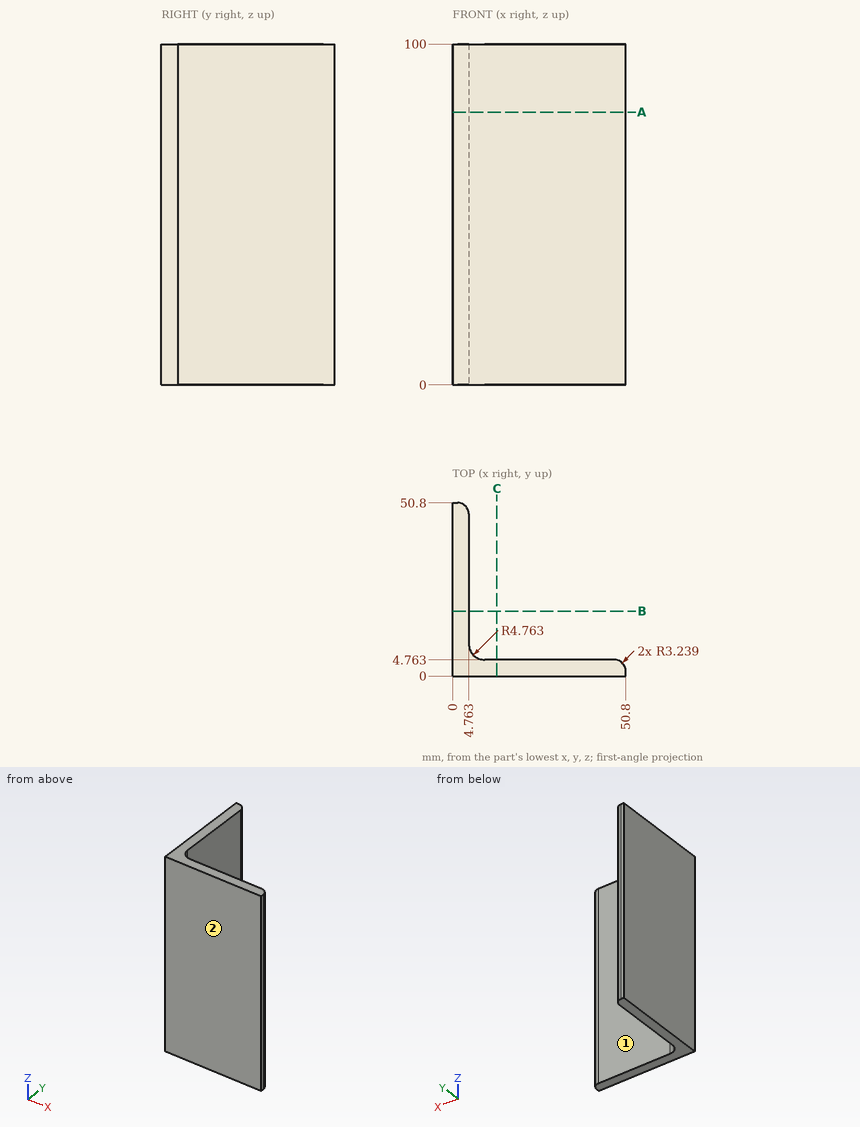
Can you work these out from the drawing? Everything is in mm from the part's minimum corner. A direction names the side the tool comes from. Round coordinates to 2 decimals unless told otherwise and drop trailing zeros. Loops run counter-clockwise (first coordinate to the right, second up) from the corner with the lowest first, then second, coordinate; pieces in that order, holes last. Notation, with made-up numbers: (-2, 33) -> (9, 33) arc R18 ccw to (9, 54) -> close; hole circle Ø1 at (13.25, 72.25). An arc over 180 degrees is marked (long way). Put each result on its own line as item: value.
Q1. Which directions (+Z, -Z, +X, -X, +Y, -Y) give clear straight access to the entire face, cutting with the end or side of a thin tool? Please do the marked faces 1 and 2.
Checks:
face 1: +Z, -Z, +X, +Y
face 2: +Z, -Z, +X, -X, -Y
Q2. Please list where these lines run through material, in increasing order: line 1 (Y direction, x = 14.5, z = 12.5); line 2 (Y direction, x = 8, z = 51). Write a range as from..to.
Checks:
line 1: 0..4.76
line 2: 0..5.01
Q3. I want a section at A-A on z = 80. Write out the boundary of the cut face in (x, y) (1 decimal).
Checks:
outline: (0, 0) -> (50.8, 0) -> (50.8, 1.5) arc R3.2 ccw to (47.6, 4.8) -> (9.5, 4.8) arc R4.8 cw to (4.8, 9.5) -> (4.8, 47.6) arc R3.2 ccw to (1.5, 50.8) -> (0, 50.8) -> close
Q4. I want a section at B-B on y = 19. Write out the boundary of the cut face in (x, z).
Checks:
outline: (0, 0) -> (4.76, 0) -> (4.76, 100) -> (0, 100) -> close
Q5. For pin 1 Ø6 at (x, z) = (14, 65.5) entering from +Y; pin 2 Ø1 at (y, z) = (14.5, 77) entering from +X; pin 3 Ø6 at (x, z) = (6, 88.5) entering from +Y (1 decimal); pin 4 Ø6 at (y, z) = (44, 39.5) entering from -X, each with a flat end and sliding along its axis, tell me the tip position at first contact or that it passes through.
Checks:
pin 1: y = 4.76
pin 2: x = 4.76
pin 3: y = 50.4
pin 4: x = 0
